```python
from build123d import *

# Parameters (mm, degrees)
SKETCH1_W           = 50
SKETCH1_H           = 15
BOSS_EXTRUDE1_DEPTH = 3
SKETCH2_R           = 2.5
CUT_EXTRUDE1_DEPTH  = 4
SKETCH3_W           = 12
SKETCH3_H           = 15
SKETCH3_W_2         = 6
SKETCH3_H_2         = 2.6
BOSS_EXTRUDE2_DEPTH = 10
SKETCH4_R           = 1.75
CUT_EXTRUDE2_DEPTH  = 16
CHAMFER1_SIZE       = 3


with BuildPart() as part:
    # Sketch1 → Boss-Extrude1 (new body)
    with BuildSketch(Plane.XY):
        with Locations((25, 7.5)):
            Rectangle(SKETCH1_W, SKETCH1_H)
    extrude(amount=BOSS_EXTRUDE1_DEPTH)

    # Sketch2 → Cut-Extrude1 (cut, through all)
    with BuildSketch(Plane.XY.offset(3)):
        with Locations((5, 7.5)):
            Circle(SKETCH2_R)
        with Locations((45, 7.5)):
            Circle(SKETCH2_R)
    extrude(amount=-CUT_EXTRUDE1_DEPTH, mode=Mode.SUBTRACT)

    # Sketch3 → Boss-Extrude2 (add)
    with BuildSketch(Plane.XY.offset(3)):
        with Locations((14.5, 7.5)):
            Rectangle(SKETCH3_W, SKETCH3_H)
        with Locations((14.5, 7.412594685)):
            Rectangle(SKETCH3_W_2, SKETCH3_H_2, mode=Mode.SUBTRACT)
        with Locations((35.5, 7.5)):
            Rectangle(SKETCH3_W, SKETCH3_H)
        with Locations((35.5, 7.412594685)):
            Rectangle(SKETCH3_W_2, SKETCH3_H_2, mode=Mode.SUBTRACT)
    extrude(amount=BOSS_EXTRUDE2_DEPTH)

    # Sketch4 → Cut-Extrude2 (cut, through all)
    with BuildSketch(Plane(origin=(0, 15, 0), x_dir=(1, 0, 0), z_dir=(0, 1, 0))):
        with Locations((35.5, -7)):
            Circle(SKETCH4_R)
        with Locations((14.5, -7)):
            Circle(SKETCH4_R)
    extrude(amount=-CUT_EXTRUDE2_DEPTH, mode=Mode.SUBTRACT)

    # Chamfer1
    chamfer1_edges = [part.edges().sort_by_distance(p)[0] for p in [
        (50, 15, 1.5),
        (50, 0, 1.5),
        (0, 0, 1.5),
        (0, 15, 1.5),
    ]]
    chamfer(chamfer1_edges, length=CHAMFER1_SIZE)


solid = part.part
```
Input: part model. Units: mm. Frame: model coordinates. A direction names the side the tool comes from. Give positions to 0.01 mm unless a question says otherwise; leave off trailing zeros. Loops run counter-clockwise (first coordinate to the right, second up) from the corner with the lowest first, then second, coordinate; pieces in that order, holes last.
1) Section query B-B on x = 5. Return the cut outline in (y, z).
A:
outline: (0, 0) - (5, 0) - (5, 3) - (0, 3) - close; (10, 0) - (15, 0) - (15, 3) - (10, 3) - close
2) Contact query for flat-ended pins moving along their axis: pin 1 (3 mm diameter, centred on y = 4, z = 7.5, fed in from -X); pin 2 (7 mm diameter, centred on x = 47, y = 11, fed in from +Z). Output: stop coordinate, or through.
A:
pin 1: stops at x = 8.5
pin 2: stops at z = 3
3) Section query A-A on y = 7.5. Return the cut outline in (x, z).
A:
outline: (0, 0) - (2.5, 0) - (2.5, 3) - (0, 3) - close; (7.5, 0) - (42.5, 0) - (42.5, 3) - (41.5, 3) - (41.5, 13) - (38.5, 13) - (38.5, 3) - (32.5, 3) - (32.5, 13) - (29.5, 13) - (29.5, 3) - (20.5, 3) - (20.5, 13) - (17.5, 13) - (17.5, 3) - (11.5, 3) - (11.5, 13) - (8.5, 13) - (8.5, 3) - (7.5, 3) - close; (47.5, 0) - (50, 0) - (50, 3) - (47.5, 3) - close
4) Line query: L1, parallel to X at y = 2.25, z = 7; L2, parallel to X at y = 10, z = 3.5; L3, parallel to Z at x = 14.5, y = 3.5. Output: solid intervals per line, ascending.
A:
L1: x = 8.5 to 12.75, 16.25 to 20.5, 29.5 to 33.75, 37.25 to 41.5
L2: x = 8.5 to 20.5, 29.5 to 41.5
L3: z = 0 to 5.25, 8.75 to 13
5) Section query D-D on y = 9.5. Return the cut outline in (x, z), and give its area (3 significant figures).
A:
outline: (0, 0) - (3.5, 0) - (3.5, 3) - (0, 3) - close; (6.5, 0) - (43.5, 0) - (43.5, 3) - (41.5, 3) - (41.5, 13) - (29.5, 13) - (29.5, 3) - (20.5, 3) - (20.5, 13) - (8.5, 13) - (8.5, 3) - (6.5, 3) - close; (46.5, 0) - (50, 0) - (50, 3) - (46.5, 3) - close; hole circle Ø3.5 at (14.5, 7); hole circle Ø3.5 at (35.5, 7)
area: 353 mm2
6) Section query C-C on z = 10. Return the cut outline in (x, y), and give its area (3 significant figures).
A:
outline: (8.5, 0) - (20.5, 0) - (20.5, 15) - (8.5, 15) - close; (29.5, 0) - (41.5, 0) - (41.5, 15) - (29.5, 15) - close; hole (11.5, 6.11) - (17.5, 6.11) - (17.5, 8.71) - (11.5, 8.71) - close; hole (32.5, 6.11) - (38.5, 6.11) - (38.5, 8.71) - (32.5, 8.71) - close
area: 329 mm2
7) Reachability of faces 1 (the flat face through (35, 7, 3)), 2 (the flat face through (41.5, 7, 8)), 3 (the flat face through (2, 8, 3)) from +Z, -Z, +X, -X, +Y, -Y: full face, straight path, thin tool, end or side. Return the list, or none.
A:
face 1: +Z
face 2: +Z, +X, +Y, -Y
face 3: +Z, -X, +Y, -Y
8) Mould query, pull axis Z, two halves, no side actions, for faces 4 (the cylindrical face through (34.11, 3.1, 8.06)), 5 (the cylindrical face through (47.31, 6.54, 1.52)), 6 (the flat face through (25, 8, 0)). Classes: released by +Z, released by -Z, zero draft, split by the parting line, or undercut.
A:
face 4: undercut
face 5: zero draft
face 6: released by -Z
